Can you work these out from the model? Positions are in its coordinate system, mm. A direction names the side the tool comes from. Round coordinates to 2 decimals unless told otherwise and drop trailing zeros. Write each loop counter-clockwise with the first axis right and the second up, starting at its lowest first coordinate (ties: lowest second). Pieces come first, ordered by that corner, then holes. Notation, with made-up numbers: M -23,6.5 L 24,6.5 A6 cw 24,10.5 Z; hole C 14.5,78 d9. An arc over 180 degrees is marked long. Answer as a JSON object with one key per item and string values. Group by question number.
1) Please list where these lines run through material, in increasing order: L1, parallel to X at y = 13.5, z = 2.5; L2, parallel to X at y = 9.5, z = -12.25; L3, parallel to Y at x = 196.5, z = -0.5. Write a range as [from, to].
2) Suppose I cut it at C-C, the plane x = 85.5. Write out the boundary of the cut face in (y, z), and give its area (3 significant figures).
3) I'm going to push flat-ended pins straight in: pin 1 Ø1 at (x, y) = (119.5, 5.5) entering from +Z; pin 2 Ø5 at (x, z) = (232, -0.5) entering from -Y; pin 3 Ø11 at (x, y) = (432, 11) entering from -Z. Where does each tip first touch, or does it pass through?
4) On a 3-axis mill with a long thin cutter (end or side, diameter ignored), from which of +Z, -Z, +X, -X, +Y, -Y can I reach the whole of each face in a straight line? I mean faces 4 (the flat face through (120, 7, 12.5)), 5 (the flat face through (115, 13, -1)), 6 (the flat face through (25, -12.3, 3.4)), 7 (the flat face through (120, 7, -12.5)). Say none if no direction works.
5) Suppose I cut it at A-A, the plane z = 0. Write out the boundary of the cut face in (x, y).
6) Suppose I cut it at B-B, the plane y = -7.75. Write out the boundary of the cut face in (x, z), and give its area (3 significant figures).
7) If we mould it in two halves opening along X, with no side actions, what happens to faces 1 (the flat face through (430, 7, -12.5)), 2 (the cylindrical face through (537.675, 0.66, 14.985)), 3 (the flat face through (0, 0, 0))? For each: +X half, -X half, draft (parallel to the pull), parting line (faces both ways), or undercut.
from build123d import *

# Parameters (mm, degrees)
SKETCH1_R           = 12.5
BOSS_EXTRUDE1_DEPTH = 550
SKETCH2_R           = 15
BOSS_EXTRUDE2_DEPTH = 25
BOSS_EXTRUDE3_START = -25
SKETCH3_R           = 15
BOSS_EXTRUDE3_DEPTH = 25
SKETCH4_W           = 10
SKETCH4_H           = 25
BOSS_EXTRUDE4_DEPTH = 15


with BuildPart() as part:
    # Sketch1 → Boss-Extrude1 (new body)
    with BuildSketch(Plane(origin=(0, 0, 0), x_dir=(0, 0, -1), z_dir=(1, 0, 0))):
        Circle(SKETCH1_R)
    extrude(amount=BOSS_EXTRUDE1_DEPTH)

    # Sketch2 → Boss-Extrude2 (add)
    with BuildSketch(Plane(origin=(550, 0, 0), x_dir=(0, 0, -1), z_dir=(1, 0, 0))):
        Circle(SKETCH2_R)
    extrude(amount=-BOSS_EXTRUDE2_DEPTH)

    # Sketch3 → Boss-Extrude3 (add)
    with BuildSketch(Plane.ZY.offset(BOSS_EXTRUDE3_START)):
        with Locations(Location((0, 0, 0), (0, 0, 180))):
            Circle(SKETCH3_R)
    extrude(amount=BOSS_EXTRUDE3_DEPTH)

    # Sketch4 → Boss-Extrude4 (add)
    with BuildSketch(Plane(origin=(0, 0, 0), x_dir=(1, 0, 0), z_dir=(0, 1, 0))):
        with Locations((120, 0)):
            Rectangle(SKETCH4_W, SKETCH4_H)
        with Locations((430, 0)):
            Rectangle(SKETCH4_W, SKETCH4_H)
    extrude(amount=BOSS_EXTRUDE4_DEPTH)


solid = part.part
Results:
{
 "1": {"L1": "[0, 25], [115, 125], [425, 435], [525, 550]", "L2": "[115, 125], [425, 435]", "L3": "[-12.49, 12.49]"},
 "2": {"outline": "C 0,0 d25", "area": "491 mm^2"},
 "3": {"pin 1": "z = 12.5", "pin 2": "y = -12.5", "pin 3": "z = -12.5"},
 "4": {"face 4": "+Z, +Y, -Y", "face 5": "+Y", "face 6": "none", "face 7": "-Z, +Y, -Y"},
 "5": {"outline": "M 0,-15 L 25,-15 L 25,-12.5 L 525,-12.5 L 525,-15 L 550,-15 L 550,15 L 525,15 L 525,12.5 L 435,12.5 L 435,15 L 425,15 L 425,12.5 L 125,12.5 L 125,15 L 115,15 L 115,12.5 L 25,12.5 L 25,15 L 0,15 Z"},
 "6": {"outline": "M 0,-12.84 L 25,-12.84 L 25,-9.81 L 525,-9.81 L 525,-12.84 L 550,-12.84 L 550,12.84 L 525,12.84 L 525,9.81 L 25,9.81 L 25,12.84 L 0,12.84 Z", "area": "11,100 mm^2"},
 "7": {"face 1": "undercut", "face 2": "draft", "face 3": "-X half"}
}
